```python
from build123d import *

# Parameters (mm, degrees)
PAD008_DEPTH        = 7
POCKET016_DEPTH     = 4
MIRROREDSKETCH012_R = 2.5
PAD009_DEPTH        = 8.3
POCKET017_DEPTH     = 2
MIRROREDSKETCH015_R = 5.5
POCKET019_DEPTH     = 0.5
SKETCH024_W         = 36.571793
SKETCH024_H         = 35.468334
POCKET022_DEPTH     = 2


with BuildPart() as part:
    # MirroredSketch010 → Pad008 (new body)
    with BuildSketch(Plane.XY.offset(-1)):
        Polygon((-4.5, 60.749919), (33.482443, 60.749919), (33.482443, 65.499919), (52.492443, 65.499919), (52.492443, 67.749919), (79.492443, 67.749919), (79.492443, 65.499919), (98.492443, 65.499919), (98.492443, 62.999919), (117.482443, 62.999919), (117.482443, 60.749919), (138.232443, 60.749919), (138.232443, -5.348885), (121.287497, -34.793261), (102.74032, -24.222717), (63.98748, -18.955575), (53.446293, -4.5), (-4.5, -4.5), align=None)
    extrude(amount=PAD008_DEPTH)

    # MirroredSketch011 → Pocket016 (cut)
    with BuildSketch(Plane.XY.offset(7)):
        Polygon((-0.5, -0.5), (-0.5, 56.75), (37.482443, 56.75), (37.482443, 61.499919), (56.492443, 61.499919), (56.492443, 63.749919), (75.492443, 63.749919), (75.492443, 61.499919), (94.492443, 61.499919), (94.492443, 58.999919), (113.482443, 58.999919), (113.482443, 56.749919), (134.232443, 56.749919), (134.232443, -4.280081), (119.807428, -29.345701), (104.047316, -20.363581), (66.215158, -15.221576), (55.48, -0.5), align=None)
    extrude(amount=-POCKET016_DEPTH, mode=Mode.SUBTRACT)

    # MirroredSketch012 → Pad009 (join)
    with BuildSketch(Plane.XY.offset(-1)):
        with Locations((18.61, 37.509997)):
            Circle(MIRROREDSKETCH012_R)
        with Locations((18.6, 18.76)):
            Circle(MIRROREDSKETCH012_R)
        with Locations((94.55, 41.252659)):
            Circle(MIRROREDSKETCH012_R)
        with Locations((61.84, 1.51)):
            Circle(MIRROREDSKETCH012_R)
        with Locations((108.3, -6.24)):
            Circle(MIRROREDSKETCH012_R)
    extrude(amount=PAD009_DEPTH)

    # MirroredSketch014 → Pocket017 (cut)
    with BuildSketch(Plane.XY.offset(6)):
        Polygon((-4.5, 60.749919), (33.482443, 60.749919), (33.482443, 65.499919), (52.492443, 65.499919), (52.492443, 67.749919), (79.492443, 67.749919), (79.492443, 65.499919), (98.492443, 65.499919), (98.492443, 62.999919), (117.482443, 62.999919), (117.482443, 60.749919), (138.232443, 60.749919), (138.232443, -5.348885), (121.287497, -34.793261), (102.74032, -24.222717), (63.98748, -18.955575), (53.446293, -4.5), (-4.5, -4.5), align=None)
        Polygon((-2.5, 58.75), (35.482443, 58.75), (35.482443, 63.499919), (54.492443, 63.499919), (54.492443, 65.749919), (77.492443, 65.749919), (77.492443, 63.499919), (96.492443, 63.499919), (96.492443, 60.999919), (115.482443, 60.999919), (115.482443, 58.749919), (136.232443, 58.749919), (136.232443, -4.814483), (120.547462, -32.069481), (103.393818, -22.293149), (65.101319, -17.088576), (54.463147, -2.5), (-2.5, -2.5), align=None, mode=Mode.SUBTRACT)
    extrude(amount=-POCKET017_DEPTH, mode=Mode.SUBTRACT)

    # MirroredSketch015 → Pocket019 (cut)
    with BuildSketch(Plane.XY.offset(-1)):
        with Locations((2.999251, 2.991994)):
            Circle(MIRROREDSKETCH015_R)
        with Locations((3, 53.216069)):
            Circle(MIRROREDSKETCH015_R)
        with Locations((130.730277, 53.25)):
            Circle(MIRROREDSKETCH015_R)
        with Locations((118.51162, -24.561471)):
            Circle(MIRROREDSKETCH015_R)
        with Locations((64.615, 31.403258)):
            Circle(MIRROREDSKETCH015_R)
    extrude(amount=POCKET019_DEPTH, mode=Mode.SUBTRACT)

    # Sketch024 → Pocket022 (cut)
    with BuildSketch(Plane.XY.offset(3)):
        with Locations((94.342338, 19.530172)):
            Rectangle(SKETCH024_W, SKETCH024_H)
    extrude(amount=-POCKET022_DEPTH, mode=Mode.SUBTRACT)


with BuildPart() as part_1:
    # Body008 placement: moved
    add(part.part.moved(Location((0, 0, -4))))


solid = part_1.part
```
Input: part model. Units: mm. Frame: model coordinates. A direction names the side the tool comes from. Coordinates: 2 decimals unless noted, no trailing zeros. Loops run counter-clockwise (first coordinate to the right, second up) from the corner with the lowest first, then second, coordinate; pieces in that order, holes last. Notation, with made-up numbers: M -38.5,-30 L -1.5,-30 A28 ccw -1.5,-3 Z; hole C -9.5,48.5 d6. An arc over 180 degrees is marked long. Use a Markdown table: item, result. Add a question column.
1) Section A-A, the plane x = 12.5. Return the cut outline in (y, z).
2) Section D-D, the plane y = -11.5. Return the cut outline in (x, z) (3 decimals).
3) Set-up query: faces 1 (the cylindrical face through (18.27, 21.24, 1.12)), 2 (the flat face through (89, 65.5, -3)), 3 (the flat face through (118, -24, -4.5)), 4 (the flat face through (84.516, -19.727, 1.014)). Return all of +Z, -Z, +X, -X, +Y, -Y with unobstructed straight access to the full face (end or side cutting, diameter ignored); none if empty.
4) Section B-B, the plane y = 18.76. Return the cut outline in (x, z), plus the area to 3 significant figures.
5) Draft query along X for faces 5 (the cylindrical face through (113.017, -24.32, -4.754)), 6 (the flat face through (62, 2, 3.3)), 7 (the flat face through (112.09, -27.25, 1.01)), 8 (the flat face through (66, 63.75, 1)). Return one class per face: +X half, -X half, draft (parallel to the pull), parting line (faces both ways), or undercut.
6) Line query: L1, parallel to X at y = 53, z = 1; L2, parallel to X at y = 35.5, z = -2.5; L3, parallel to Y at x = 3, z = 0.5. Output: solid intervals per line, ascending. Write a range as from..to.
7) Pin query (flat end, axial travel): P1, Ø1.5, axis at x = 41, z = 1, coming from the +Y side; P2, Ø4, axis at x = 125, z = -1.5, coming from the +Y side; P3, Ø3.5, axis at x = 128, z = 0.5, coming from the -Y side. Return the tip coordinate at first contact, or that it passes through.
8) Section C-C, the plane x = 108.3. Return the cut outline in (y, z).
Answer below:
| question | item | result |
|---|---|---|
| 1 | outline | M -4.5,-5 L 60.75,-5 L 60.75,0 L 58.75,0 L 58.75,2 L 56.75,2 L 56.75,-1 L -0.5,-1 L -0.5,2 L -2.5,2 L -2.5,0 L -4.5,0 Z |
| 2 | outline | M 58.551,-5 L 134.693,-5 L 134.693,0 L 132.385,0 L 132.385,2 L 130.077,2 L 130.077,-1 L 63.501,-1 L 63.501,2 L 61.026,2 L 61.026,0 L 58.551,0 Z |
| 3 | face 1 | +Z |
| 3 | face 2 | +Z, -Z, +X, +Y |
| 3 | face 3 | -Z |
| 3 | face 4 | +Z, -X, -Y |
| 4 | outline | M -4.5,-5 L 138.23,-5 L 138.23,0 L 136.23,0 L 136.23,2 L 134.23,2 L 134.23,-1 L 112.63,-1 L 112.63,-3 L 76.06,-3 L 76.06,-1 L 21.1,-1 L 21.1,3.3 L 16.1,3.3 L 16.1,-1 L -0.5,-1 L -0.5,2 L -2.5,2 L -2.5,0 L -4.5,0 Z |
| 4 | area | 535 mm2 |
| 5 | face 5 | undercut |
| 5 | face 6 | draft |
| 5 | face 7 | -X half |
| 5 | face 8 | undercut |
| 6 | L1 | -2.5..-0.5, 134.23..136.23 |
| 6 | L2 | -4.5..76.06, 112.63..138.23 |
| 6 | L3 | -2.5..-0.5, 56.75..58.75 |
| 7 | P1 | y = 63.5 |
| 7 | P2 | y = 60.75 |
| 7 | P3 | y = -26.04 |
| 8 | outline | M -27.39,-5 L 63,-5 L 63,0 L 61,0 L 61,2 L 59,2 L 59,-1 L 37.26,-1 L 37.26,-3 L 1.8,-3 L 1.8,-1 L -3.74,-1 L -3.74,3.3 L -8.74,3.3 L -8.74,-1 L -22.79,-1 L -22.79,2 L -25.09,2 L -25.09,0 L -27.39,0 Z |
